Autodesk Inventor part; units mm, degrees
ref_plane "YZ Plane" through (0, 0, 0) normal (1, 0, 0) x (0, 1, 0)
ref_plane "XZ Plane" through (0, 0, 0) normal (0, 1, 0) x (-1, 0, 0)
ref_plane "XY Plane" through (0, 0, 0) normal (0, 0, 1) x (1, 0, 0)
sketch "Sketch1" plane through (0, 0, 0) normal (1, 0, 0) x (0, 1, 0)
  line L0 (-12.5, 10) -> (12.5, 10)
  line L1 (12.5, 10) -> (12.5, -10)
  line L2 (12.5, -10) -> (-12.5, -10)
  line L3 (-12.5, -10) -> (-12.5, 10)
  line L4 (-12.5, 10) -> (12.5, -10) construction
  line L5 (12.5, 10) -> (-12.5, -10) construction
  line L6 (5, 10) -> (-5, 10)
  line L7 (-5, 10) -> (-5, 13)
  line L8 (-5, 13) -> (5, 13)
  line L9 (5, 13) -> (5, 10)
  line L10 (-12.5, 5) -> (-15.5, 5)
  line L11 (-15.5, 5) -> (-15.5, -5)
  line L12 (-15.5, -5) -> (-12.5, -5)
  line L13 (-12.5, -5) -> (-12.5, 5)
  circle A0 centre (0, -10) radius 10
  point P0 (0, 0)
  point P1 (0, 13)
  point P2 (0, 0)
  dimension "d0" = 25
  dimension "d1" = 20
  dimension "d2" = 10
  dimension "d3" = 3
  dimension "d4" = 3
  dimension "d5" = 10
  dimension "d8" = 5
extrude "Extrusion1" add sketch "Sketch1" along normal blind 3 contours L0 L1 L2 A0 L3 | L7 L8 L9 L0 | L3 L12 L11 L10 | A0 L2 picked at (-0.8971, -4.5365)
properties part number "Back support"
Can you work these out from the model? Positions are in its coordinate system, mm. A direction names the side the tool comes from. Round coordinates to 2 decimals unless told otherwise and drop trailing zeros. Loops run counter-clockwise (first coordinate to the right, second up) from the corner with the lowest first, then second, coordinate; pieces in that order, holes last. Notation, with made-up numbers: M 54,61 L 97,61 A28 cw 97,97 Z; hole C 39.5,11 d7. An arc over 180 degrees is marked long. Write item = value, one per line. Start each with the question number.
(1) Suppose I cut it at A-A on x = 2.1. Write out the boundary of the cut face in (y, z).
(2) Which directions (+Z, -Z, +X, -X, +Y, -Y) give clear straight access to the entire face, cutting with the end or side of a thin tool? Please do faces 1 (the face through (1, 5, 12)), 2 (the face through (1, -9, 10)), 3 (the face through (1, 0, -10)), 4 (the face through (1, -14, -5)).
(3) I'm going to push flat-ended pins straight in: P1, Ø1.5, axis at x = 1, y = -14.5, coming from the +Z side; P2, Ø0.9, axis at x = 1.5, z = 6.5, coming from the -Y side; P3, Ø1.5, axis at x = 2, y = 10.5, coming from the +Z side; P4, Ø5, axis at y = -9.5, z = -7.5, coming from the -X side. Where does each tip first touch, or does it pass through?
(4) Suppose I cut it at B-B on z = -8. Write out the boundary of the cut face in (x, y).
(5) Suppose I cut it at C-C on y = -12. Write out the boundary of the cut face in (x, z), plus the area to 3 significant figures.
(6) I need wall thicknesses on line 1 along Z through (x, y) = (0.2, -7); line 2 along Y through (x, z) = (1.9, 5.75); line 3 along Y through (x, z) = (1.4, 10.75). Which ranges of each line are inside material? Lowest first, please.
Answer block:
q1.outline = M -15.5,-5 L -12.5,-5 L -12.5,-10 L 12.5,-10 L 12.5,10 L 5,10 L 5,13 L -5,13 L -5,10 L -12.5,10 L -12.5,5 L -15.5,5 Z
q2.face_1 = +Z, +X, -X, +Y
q2.face_2 = +Z, +X, -X, -Y
q2.face_3 = -Z, +X, -X, +Y, -Y
q2.face_4 = -Z, +X, -X, -Y
q3.P1 = 5
q3.P2 = -12.5
q3.P3 = 10
q3.P4 = 0
q4.outline = M 0,-12.5 L 3,-12.5 L 3,12.5 L 0,12.5 Z
q5.outline = M 0,-10 L 3,-10 L 3,10 L 0,10 Z
q5.area = 60.0 mm²
q6.line_1 = -10 to 10
q6.line_2 = -12.5 to 12.5
q6.line_3 = -5 to 5
